```python
from build123d import *

# Parameters (mm, degrees)
SKETCH1_W             = 15
SKETCH1_H             = 40
SKETCH1_R             = 2
BOSS_EXTRUDE1_DEPTH   = 30
BOSS_EXTRUDE1_2_DEPTH = 30
BOSS_EXTRUDE2_DEPTH   = 5
SKETCH3_W             = 25
SKETCH3_H             = 25
CUT_EXTRUDE1_DEPTH    = 25


with BuildPart() as part:
    # Sketch1 → Boss-Extrude1 (new body)
    with BuildSketch(Plane(origin=(0, 0, 0), x_dir=(1, 0, 0), z_dir=(0, 1, 0))):
        with Locations((7.5, 20)):
            Rectangle(SKETCH1_W, SKETCH1_H)
        with Locations(Location((3.75, 35, 0), (0, 0, 90))):
            Circle(SKETCH1_R, mode=Mode.SUBTRACT)
        with Locations(Location((11.25, 35, 0), (0, 0, 270))):
            Circle(SKETCH1_R, mode=Mode.SUBTRACT)
        with Locations(Location((11.25, 5, 0), (0, 0, 90))):
            Circle(SKETCH1_R, mode=Mode.SUBTRACT)
        with Locations(Location((3.75, 5, 0), (0, 0, 270))):
            Circle(SKETCH1_R, mode=Mode.SUBTRACT)
    extrude(amount=BOSS_EXTRUDE1_DEPTH)



with BuildPart() as body_2:
    # Sketch1 → Boss-Extrude1 2 (new body)
    with BuildSketch(Plane(origin=(0, 0, 0), x_dir=(1, 0, 0), z_dir=(0, 1, 0))):
        with Locations((147.93, 20)):
            Rectangle(SKETCH1_W, SKETCH1_H)
        with Locations(Location((144.18, 5, 0), (0, 0, 270))):
            Circle(SKETCH1_R, mode=Mode.SUBTRACT)
        with Locations(Location((151.68, 5, 0), (0, 0, 90))):
            Circle(SKETCH1_R, mode=Mode.SUBTRACT)
        with Locations(Location((151.68, 35, 0), (0, 0, 270))):
            Circle(SKETCH1_R, mode=Mode.SUBTRACT)
        with Locations(Location((144.18, 35, 0), (0, 0, 90))):
            Circle(SKETCH1_R, mode=Mode.SUBTRACT)
    extrude(amount=BOSS_EXTRUDE1_2_DEPTH)


with BuildPart() as part_1:
    add(part.part)

    add(body_2.part)  # Boss-Extrude2 merges body 2
    # Sketch2 → Boss-Extrude2 (add)
    with BuildSketch(Plane(origin=(0, 30, 0), x_dir=(1, 0, 0), z_dir=(0, 1, 0))):
        Polygon((130.586527376, -27.5), (24.843472624, -27.5), (0, -7.089654433), (0, 47.089654433), (24.843472624, 67.5), (130.586527376, 67.5), (155.43, 47.089654433), (155.43, -7.089654433), align=None)
        Polygon((15, 40), (30.215, 52.5), (125.215, 52.5), (140.43, 40), (140.43, 0), (125.215, -12.5), (30.215, -12.5), (15, 0), align=None, mode=Mode.SUBTRACT)
    extrude(amount=BOSS_EXTRUDE2_DEPTH)

    # Sketch3 → Cut-Extrude1 (cut)
    with BuildSketch(Plane(origin=(15, 0, 0), x_dir=(0, 0, -1), z_dir=(1, 0, 0))):
        with Locations((20, 17.5)):
            Rectangle(SKETCH3_W, SKETCH3_H)
    extrude(amount=-CUT_EXTRUDE1_DEPTH, mode=Mode.SUBTRACT)


solid = part_1.part
```
Geometry check sheet. Reference: the model listing, model coordinates, mm. A direction names the side the tool comes from. Give positions to 0.01 mm unless a question says otherwise; leave off trailing zeros. Write each loop counter-clockwise with the first axis right and the second up, starting at its lowest first coordinate (ties: lowest second). Pieces come first, ordered by that corner, then holes.
1) Material ranges on L1, parallel to Z at x = 144.18, y = 7.25; L2, parallel to Z at x = 11, y = 20; L3, parallel to X at y = 19.75, z = -35, recorded low to high.
2) Section check D-D, the plane z = -5. Record the boundary of the cut face in (x, y), and give its area (3 significant figures).
3) Section check C-C, the plane x = 121. Record the boundary of the cut face in (y, z).
4) Section check A-A, the plane y = 16. State how many separate pieces and enclosed holes the cut face has, and give its area (3 significant figures).
5) Release check for a two-part mould opening along Z. For faces 6 (the flat face through (148, 0, -20)), 7 (the flat face through (152, 30, -5)), 8 (the flat face through (142.83, 32.47, -57.44)) record: pulls with the +Z half, pulls with the -Z half, needs draft (parallel to the pull), parting line crosses it, or undercut.
6) Section check B-B, the plane z = -17.5. Record the boundary of the cut face in (x, y).
7) Access from +Z, -Z, +X, -X, +Y, -Y to the whole of each face (thin tool, end or side, straight path). Record for faces 1 (the cylindrical face through (9.898, 14.79, -3.526)), 2 (the flat face through (132.716, 32.465, -46.338)), 3 (the flat face through (155.43, 17, -20)), 4 (the flat face through (79, 30, -57)), 5 (the flat face through (79, 30, 17)).
8) Gauge pin test, flat ends, axial feed: pin 1 (1.2 mm diameter, centred on x = 4, z = -5, fed in from -Y); pin 2 (4.5 mm diameter, centred on x = 3.75, z = -5, fed in from -Y); pin 3 (12 mm diameter, centred on x = 145, y = 17.5, fed in from +Z). Record the tip position at first contact, or that the pin passes through.
Computed:
1. L1: z = -40 to -37, -33 to -7, -3 to 0
1. L2: z = -40 to -36.98, -33.02 to -32.5, -7.5 to -6.98, -3.02 to 0
1. L3: x = 0 to 1.75, 5.75 to 9.25, 13.25 to 15, 140.43 to 142.18, 146.18 to 149.68, 153.68 to 155.43
2. outline: (0, 0) - (1.75, 0) - (1.75, 30) - (5.75, 30) - (5.75, 0) - (9.25, 0) - (9.25, 30) - (13.25, 30) - (13.25, 0) - (15, 0) - (15, 35) - (0, 35) - close; (140.43, 0) - (142.18, 0) - (142.18, 30) - (146.18, 30) - (146.18, 0) - (149.68, 0) - (149.68, 30) - (153.68, 30) - (153.68, 0) - (155.43, 0) - (155.43, 35) - (140.43, 35) - close
2. area: 570 mm2
3. outline: (30, -67.5) - (35, -67.5) - (35, -52.5) - (30, -52.5) - close; (30, 12.5) - (35, 12.5) - (35, 27.5) - (30, 27.5) - close
4. separate pieces: 3
4. enclosed holes: 8
4. area: 724 mm2
5. face 6: needs draft
5. face 7: undercut
5. face 8: pulls with the -Z half
6. outline: (0, 0) - (15, 0) - (15, 5) - (0, 5) - close; (0, 30) - (15, 30) - (15, 35) - (0, 35) - close; (140.43, 0) - (155.43, 0) - (155.43, 35) - (140.43, 35) - close
7. face 1: -Y
7. face 2: +Y, -Y
7. face 3: +Z, -Z, +X, +Y, -Y
7. face 4: -Z, +X, -X, -Y
7. face 5: +Z, +X, -X, -Y
8. pin 1: stops at y = 30
8. pin 2: stops at y = 0
8. pin 3: stops at z = 0
